CAD build for the part. Positions are in the model's coordinates, mm. A direction names the side the tool comes from. Give positions to 0.01 mm unless a question says otherwise; leave off trailing zeros. Order: outer loops, then holes, each group sorted by start corner. A loop starts at its lowest first (then second) coordinate and runs counter-clockwise, first axis right, second up.
from build123d import *

# Parameters (mm, degrees)
BOSS_EXTRUDE1_DEPTH = 1.2
SKETCH2_R           = 3.5
BOSS_EXTRUDE2_DEPTH = 2.1
SKETCH3_R           = 2.5
CUT_EXTRUDE1_DEPTH  = 1
SKETCH4_R           = 1
CUT_EXTRUDE2_DEPTH  = 19.149516235
SKETCH6_R           = 2.45
CUT_EXTRUDE3_DEPTH  = 2.1
SKETCH7_R           = 0.5
CUT_EXTRUDE4_DEPTH  = 19.303140156
SKETCH8_R           = 0.5
CUT_EXTRUDE5_DEPTH  = 19.303140156
CUT_EXTRUDE6_DEPTH  = 10


with BuildPart() as part:
    # Sketch1 → Boss-Extrude1 (new body)
    with BuildSketch(Plane.XY):
        with BuildLine():
            Line((-2, -6.75), (-2, -3))
            Line((-2, -3), (-14, -1.9))
            ThreePointArc((-14, -1.9), (-15.733799273, 0), (-14, 1.9))
            Line((-14, 1.9), (-2, 3))
            Line((-2, 3), (-2, 6.75))
            ThreePointArc((-2, 6.75), (0, 8.75), (2, 6.75))
            Line((2, 6.75), (2, 3))
            Line((2, 3), (14, 1.9))
            ThreePointArc((14, 1.9), (15.733799273, 0), (14, -1.9))
            Line((14, -1.9), (2, -3))
            Line((2, -3), (2, -6.75))
            ThreePointArc((2, -6.75), (0, -8.75), (-2, -6.75))
        make_face()
    extrude(amount=BOSS_EXTRUDE1_DEPTH)

    # Sketch2 → Boss-Extrude2 (add)
    with BuildSketch(Plane(origin=(0, 0, 0), x_dir=(-1, 0, 0), z_dir=(0, 0, -1))):
        Circle(SKETCH2_R)
    extrude(amount=BOSS_EXTRUDE2_DEPTH)

    # Sketch3 → Cut-Extrude1 (cut)
    with BuildSketch(Plane.XY.offset(1.2)):
        Circle(SKETCH3_R)
    extrude(amount=-CUT_EXTRUDE1_DEPTH, mode=Mode.SUBTRACT)

    # Sketch4 → Cut-Extrude2 (cut, through all)
    with BuildSketch(Plane.XY.offset(0.2)):
        Circle(SKETCH4_R)
    extrude(amount=-CUT_EXTRUDE2_DEPTH, mode=Mode.SUBTRACT)

    # Sketch6 → Cut-Extrude3 (cut)
    with BuildSketch(Plane(origin=(0, 0, -2.1), x_dir=(-1, 0, 0), z_dir=(0, 0, -1))):
        Circle(SKETCH6_R)
    extrude(amount=-CUT_EXTRUDE3_DEPTH, mode=Mode.SUBTRACT)

    # Sketch7 → Cut-Extrude4 (cut, through all)
    with BuildSketch(Plane.XY.offset(1.2)):
        with Locations((0, -4.5)):
            Circle(SKETCH7_R)
        with Locations((0, -6.5)):
            Circle(SKETCH7_R)
        with Locations((0, 4.5)):
            Circle(SKETCH7_R)
        with Locations((0, 6.5)):
            Circle(SKETCH7_R)
    extrude(amount=-CUT_EXTRUDE4_DEPTH, mode=Mode.SUBTRACT)

    # Sketch8 → Cut-Extrude5 (cut, through all)
    with BuildSketch(Plane.XY.offset(1.2)):
        with Locations((-4.5, 0)):
            Circle(SKETCH8_R)
        with Locations((-6.5, 0)):
            Circle(SKETCH8_R)
        with Locations((-8.5, 0)):
            Circle(SKETCH8_R)
        with Locations((-10.5, 0)):
            Circle(SKETCH8_R)
        with Locations((-12.5, 0)):
            Circle(SKETCH8_R)
        with Locations((-14.5, 0)):
            Circle(SKETCH8_R)
        with Locations(Location((4.5, 0, 0), (0, 0, 180))):
            Circle(SKETCH8_R)
        with Locations(Location((6.5, 0, 0), (0, 0, 180))):
            Circle(SKETCH8_R)
        with Locations(Location((8.5, 0, 0), (0, 0, 180))):
            Circle(SKETCH8_R)
        with Locations(Location((10.5, 0, 0), (0, 0, 180))):
            Circle(SKETCH8_R)
        with Locations(Location((12.5, 0, 0), (0, 0, 180))):
            Circle(SKETCH8_R)
        with Locations(Location((14.5, 0, 0), (0, 0, 180))):
            Circle(SKETCH8_R)
    extrude(amount=-CUT_EXTRUDE5_DEPTH, mode=Mode.SUBTRACT)

    # Sketch10 → Cut-Extrude6 (cut)
    with BuildSketch(Plane(origin=(0, 0, 0), x_dir=(-1, 0, 0), z_dir=(0, 0, -1))):
        with BuildLine():
            Line((-2, 3), (-3.5, 8.058048999))
            Line((-3.5, 8.058048999), (0.410688034, 10.263711762))
            Line((0.410688034, 10.263711762), (4.972399658, 6.328608878))
            Line((4.972399658, 6.328608878), (2, 3))
            ThreePointArc((2, 3), (0, 3.605551275), (-2, 3))
        make_face()
        with BuildLine():
            Line((-2, -3), (-3.79905406, -6.652770289))
            Line((-3.79905406, -6.652770289), (-0.630835306, -10.284036399))
            Line((-0.630835306, -10.284036399), (2.565835598, -9.787591171))
            Line((2.565835598, -9.787591171), (3.731558209, -4.826385145))
            Line((3.731558209, -4.826385145), (2, -3))
            ThreePointArc((2, -3), (0, -3.605551275), (-2, -3))
        make_face()
    extrude(amount=-CUT_EXTRUDE6_DEPTH, mode=Mode.SUBTRACT)


solid = part.part
1. Mould opens along X. For faces 3 (the flat face through (-1, -1, 0)), 4 (the cylindrical face through (-15.733, -0.04, 0.592)), 5 (the flat face through (7.916, 2.458, 0.592)) say: released by +X, released by -X, zero draft, split by the parting line, or undercut.
2. Saw through at C-C on y = 1.5. Give the cut face in (x, z).
3. 3-axis set-ups, long thin cutter, end or side, ignore diameter. For faces 1 (the cylindrical face through (0.5, -2.4, -1.1)), 2 (the cylindrical face through (-8, 0, 1)): which of +Z, -Z, +X, -X, +Y, -Y reach the whole face in a straight line?
4. Saw through at A-A on x = -12.5. Give the cut face in (y, z).
5. Wall check: line 1 (Z direction, x = -14, y = 0.25); line 2 (X direction, y = 0.25, z = -0.9); line 3 (X direction, y = 1.25, z = 0.25). Give the ranges that are in metal, low to high.
6. Pin check, flat tips, straight feed: P1, Ø4, axis at x = 0, y = 0, coming from the -Z side; P2, Ø3, axis at x = 0, y = 0, coming from the +Z side; P3, Ø1, axis at y = 2, z = 0.5, coming from the -X side; P4, Ø4, axis at x = -0.5, y = -0.5, coming from the +Z side. Stop position of each tip, or through.
7. Saw through at D-D on x = -6.5. Give the cut face in (y, z).
8. Saw through at B-B on z = -0.8. Give the cut face in (x, y).
Reported:
1. face 3: undercut
1. face 4: released by -X
1. face 5: released by +X
2. outline: (-15, 0) - (-3.16, 0) - (-3.16, -2.1) - (-1.94, -2.1) - (-1.94, 0) - (1.94, 0) - (1.94, -2.1) - (3.16, -2.1) - (3.16, 0) - (15, 0) - (15, 1.2) - (2, 1.2) - (2, 0.2) - (-2, 0.2) - (-2, 1.2) - (-15, 1.2) - close
3. face 1: -Z
3. face 2: +Z, -Z
4. outline: (-2.04, 0) - (-0.5, 0) - (-0.5, 1.2) - (-2.04, 1.2) - close; (0.5, 0) - (2.04, 0) - (2.04, 1.2) - (0.5, 1.2) - close
5. line 1: z = 0 to 1.2
5. line 2: x = -3.49 to -2.44, 2.44 to 3.49
5. line 3: x = -15.27 to -2.17, 2.17 to 15.27
6. P1: stops at z = 0
6. P2: stops at z = 0.2
6. P3: stops at x = -15
6. P4: stops at z = 1.2
7. outline: (-2.59, 0) - (-0.5, 0) - (-0.5, 1.2) - (-2.59, 1.2) - close; (0.5, 0) - (2.59, 0) - (2.59, 1.2) - (0.5, 1.2) - close
8. outline: circle Ø7 at (0, 0); hole circle Ø4.9 at (0, 0)
